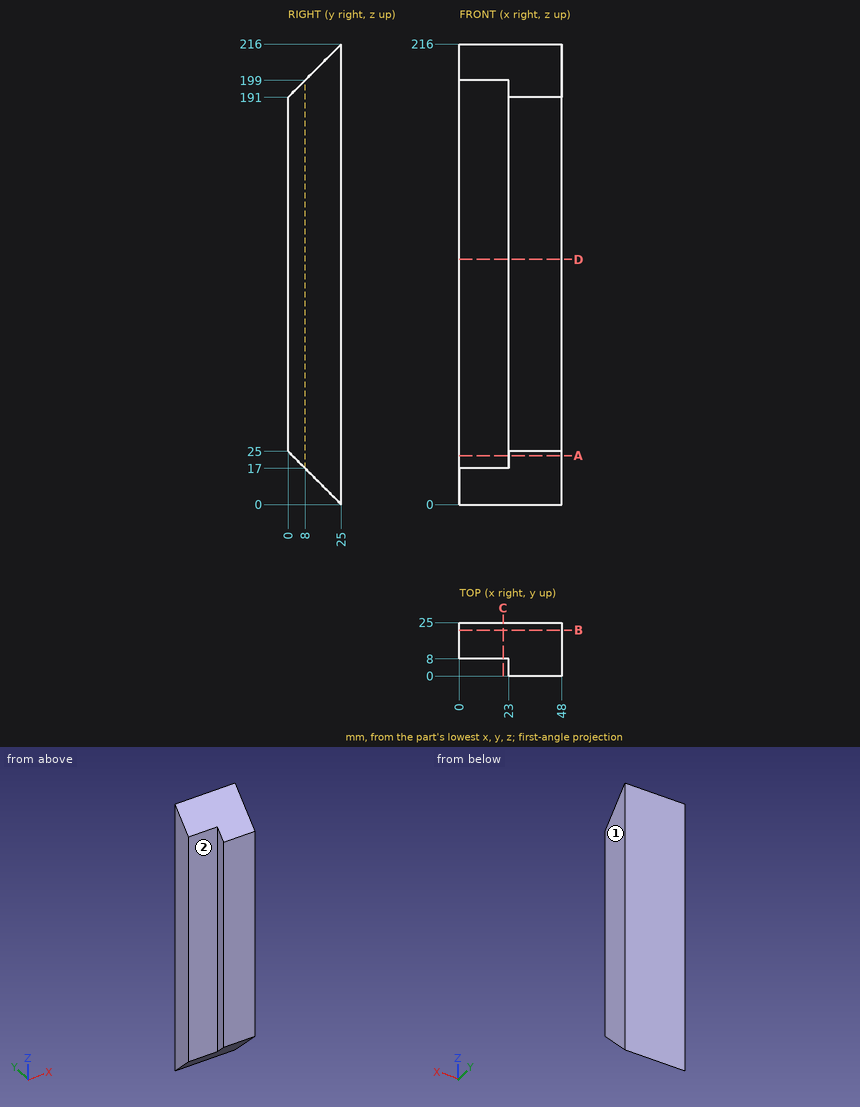
Input: dimensioned drawing with shaded views. Units: mm. Origin: part minimum x, y, z. A direction names the side the tool comes from. Give positions to 0.01 mm unless a question says otherwise; leave off trailing zeros. Write each loop counter-clockwise with the first axis right and the second up, starting at its lowest first coordinate (ties: lowest second). Pieces come first, ordered by that corner, then holes.
1. Section query D-D, the plane z = 115. Return loops of the section in (x, y).
2. Section query C-C, the plane x = 20.5. Return loops of the section in (y, z), then the cut area to 3 significant figures.
3. Reachability of the marked faces 1 and 2 from +Z, -Z, +X, -X, +Y, -Y: full face, straight path, thin tool, end or side. Return the list, or none.
4. Section query A-A, the plane z = 23. Return loops of the section in (x, y).
5. Section query B-B, the plane y = 21.5. Return loops of the section in (x, z).
6. Line query: probe 1 along Y at (x, z) = (17, 40); probe 2 along X at (y, z) = (4, 98.5); probe 3 along Z at (x, y) = (9.5, 22.5). Output: solid intervals per line, ascending.
7. Pin query (flat end, axial travel): P1, Ø5, axis at x = 12, y = 20, coming from the -Z side; P2, Ø4, axis at y = 4, z = 102, coming from the -X side; P3, Ø10, axis at x = 24, y = 10, coming from the -Z side. Return the tip coordinate at first contact, or that it passes through.
Computed:
1. outline: (0, 8) - (23, 8) - (23, 0) - (48, 0) - (48, 25) - (0, 25) - close
2. outline: (8, 17) - (25, 0) - (25, 216) - (8, 199) - close
2. area: 3,380 mm2
3. face 1: +Z, -Z, +X, +Y, -Y
3. face 2: +Z, -Z, -X, -Y
4. outline: (0, 8) - (23, 8) - (23, 2) - (48, 2) - (48, 25) - (0, 25) - close
5. outline: (0, 3.5) - (48, 3.5) - (48, 212.5) - (0, 212.5) - close
6. probe 1: y = 8 to 25
6. probe 2: x = 23 to 48
6. probe 3: z = 2.5 to 213.5
7. P1: stops at z = 2.5
7. P2: stops at x = 23
7. P3: stops at z = 10
